```python
from build123d import *

# Parameters (mm, degrees)
ESQUISSE1_W                                    = 32
ESQUISSE1_H                                    = 18
BOSS_EXTRU_1_DEPTH                             = 2
ESQUISSE2_W                                    = 19
ESQUISSE2_H                                    = 12
BOSS_EXTRU_2_DEPTH                             = 1.4
CONG_1_R                                       = 1
CONG_2_R                                       = 0.6
CONG_3_R                                       = 1
FRAISAGE_POUR_VIS_T_TE_FRAIS_E_M21_D           = 2.6
FRAISAGE_POUR_VIS_T_TE_FRAIS_E_M21_CSINK_D     = 4.4
FRAISAGE_POUR_VIS_T_TE_FRAIS_E_M21_CSINK_ANGLE = 90


with BuildPart() as part:
    # Esquisse1 → Boss.-Extru.1 (new body)
    with BuildSketch(Plane.XY):
        Rectangle(ESQUISSE1_W, ESQUISSE1_H)
    extrude(amount=BOSS_EXTRU_1_DEPTH)

    # Esquisse2 → Boss.-Extru.2 (add)
    with BuildSketch(Plane(origin=(0, 0, 0), x_dir=(-1, 0, 0), z_dir=(0, 0, -1))):
        Rectangle(ESQUISSE2_W, ESQUISSE2_H)
    extrude(amount=BOSS_EXTRU_2_DEPTH)

    # Congé1
    cong_1_edges = [part.edges().sort_by_distance(p)[0] for p in [
        (16, -9, 1),
        (-16, -9, 1),
        (-16, 9, 1),
        (16, 9, 1),
    ]]
    fillet(cong_1_edges, radius=CONG_1_R)

    # Congé2
    cong_2_edges = [part.edges().sort_by_distance(p)[0] for p in [
        (16, 0, 2),
        (0, -9, 2),
        (0, 9, 2),
        (-16, 0, 2),
        (15.707106781, 8.707106781, 2),
        (-15.707106781, 8.707106781, 2),
        (-15.707106781, -8.707106781, 2),
        (15.707106781, -8.707106781, 2),
    ]]
    fillet(cong_2_edges, radius=CONG_2_R)

    # Congé3
    cong_3_edges = [part.edges().sort_by_distance(p)[0] for p in [
        (-9.5, -6, -0.7),
        (-9.5, 6, -0.7),
        (9.5, 6, -0.7),
        (9.5, -6, -0.7),
    ]]
    fillet(cong_3_edges, radius=CONG_3_R)

    # Fraisage pour vis à tête fraisée M21 (through all)
    with Locations(Plane.XY.offset(2)):
        with Locations((-13, 0)):
            fraisage_pour_vis_t_te_frais_e_m21 = CounterSinkHole(FRAISAGE_POUR_VIS_T_TE_FRAIS_E_M21_D / 2, FRAISAGE_POUR_VIS_T_TE_FRAIS_E_M21_CSINK_D / 2, counter_sink_angle=FRAISAGE_POUR_VIS_T_TE_FRAIS_E_M21_CSINK_ANGLE)

    # Symétrie1: Fraisage pour vis à tête fraisée M21 across plane
    add(fraisage_pour_vis_t_te_frais_e_m21.mirror(Plane(origin=(0, 0, 0), x_dir=(0, 0, 1), z_dir=(1, 0, 0))), mode=Mode.SUBTRACT)


solid = part.part
```
Could you check a few things on this model? Use its own coordinates, in mm. A direction names the side the tool comes from. Coordinates: 2 decimals unless noted, no trailing zeros. Write each loop counter-clockwise with the first axis right and the second up, starting at its lowest first coordinate (ties: lowest second). Pieces come first, ordered by that corner, then holes. Notation, with made-up numbers: (-3.5, 85) -> (12.5, 85) arc R27 cw to (12.5, 110) -> close; hole circle Ø6 at (85.25, -13). An arc over 180 degrees is marked (long way). One line per question, with ' | ' between items. Start each with the question number.
1. If we section it at C-C (z = 0.4): Please give me the cut outline in (x, y), and give its area (3 significant figures).
2. If we section it at A-A (y = 0): Please give me the cut outline in (x, z).
3. For faces 1 (the face through (9.5, 0, -1)), 2 (the face through (9.215, -5.699, -0.71)), 3 (the face through (0, -6, -1)), which set-ups out of +Z, -Z, +X, -X, +Y, -Y let a thin tool reach every point of the face, with its end or its side?
4. Please list where these lines run through material, in increasing order: line 1 along X through (y, z) = (0, 0.85); line 2 along Y through (x, z) = (13, 0.75); line 3 along Z through (x, y) = (13.5, -4.5).
5. Thinking about a two-plate mould opening in X: for faces 4 (the face through (-9.5, 0, -1)), 5 (the face through (9.215, 5.699, -0.71)), 6 (the face through (11.7, 0.06, 0.54)), which applies, pulls with the +X half, pulls with the -X half, needs draft (parallel to the pull), parting line crosses it, or undercut?
6. If we section it at D-D (x = -4): Please give me the cut outline in (y, z).
7. Will these pins go through, and if not, where does the flat tip stop? P1, Ø4, axis at x = -13, y = 0, coming from the +Z side; P2, Ø1.1, axis at x = 1, z = -0.5, coming from the +Y side; P3, Ø1.5, axis at x = -3, z = -1, coming from the -Y side.
8. If we section it at B-B (x = -13): Please give me the cut outline in (y, z), and give its area (3 significant figures).
Return value:
1) outline: (-16, -8) arc R1 ccw to (-15, -9) -> (15, -9) arc R1 ccw to (16, -8) -> (16, 8) arc R1 ccw to (15, 9) -> (-15, 9) arc R1 ccw to (-16, 8) -> close; hole circle Ø2.6 at (-13, 0); hole circle Ø2.6 at (13, 0) | area: 565 mm²
2) outline: (-16, 0) -> (-14.3, 0) -> (-14.3, 1.1) -> (-15.2, 2) -> (-15.4, 2) arc R0.6 ccw to (-16, 1.4) -> close; (-11.7, 0) -> (-9.5, 0) -> (-9.5, -1.4) -> (9.5, -1.4) -> (9.5, 0) -> (11.7, 0) -> (11.7, 1.1) -> (10.8, 2) -> (-10.8, 2) -> (-11.7, 1.1) -> close; (14.3, 0) -> (16, 0) -> (16, 1.4) arc R0.6 ccw to (15.4, 2) -> (15.2, 2) -> (14.3, 1.1) -> close
3) face 1: -Z, +X, +Y, -Y | face 2: -Z, +X, -Y | face 3: -Z, +X, -X, -Y
4) line 1: x = -16 to -14.3, -11.7 to 11.7, 14.3 to 16 | line 2: y = -9 to -1.3, 1.3 to 9 | line 3: z = 0 to 2
5) face 4: pulls with the -X half | face 5: pulls with the +X half | face 6: undercut
6) outline: (-9, 0) -> (-6, 0) -> (-6, -1.4) -> (6, -1.4) -> (6, 0) -> (9, 0) -> (9, 1.4) arc R0.6 ccw to (8.4, 2) -> (-8.4, 2) arc R0.6 ccw to (-9, 1.4) -> close
7) P1: stops at z = 1.8 | P2: stops at y = 9 | P3: stops at y = -6
8) outline: (-9, 0) -> (-1.3, 0) -> (-1.3, 1.1) -> (-2.2, 2) -> (-8.4, 2) arc R0.6 ccw to (-9, 1.4) -> close; (1.3, 0) -> (9, 0) -> (9, 1.4) arc R0.6 ccw to (8.4, 2) -> (2.2, 2) -> (1.3, 1.1) -> close | area: 29.8 mm²
